from build123d import *

# Parameters (mm, degrees)
F1_DEPTH = 12.7
F2_DEPTH = 13.0175
F3_DEPTH = 12.065
F4_DEPTH = 13.0175
F5_DEPTH = 13.0175
F6_DEPTH = 12.7


with BuildPart() as f1:
    # F0 (on Front) → F1 (new body, symmetric)
    with BuildSketch(Plane.XZ):
        Polygon((28.078623, 2.014946), (28.042302, 12.433615), (27.101992, 12.433615), (27.101992, 12.053489), (26.661847, 12.053489), (26.661847, 12.433615), (22.280401, 12.433615), (20.983042, 11.892567), (21.152996, 9.532103), (23.8156, 7.73815), (23.8156, 6.359639), (23.060251, 5.60429), (23.060251, 2.620663), (24.042204, 2.035267), (24.042204, -0.005739), (25.287887, 0), (25.434768, 0.933369), (26.649874, 1.414069), (26.649874, 1.707831), (27.103869, 1.707831), (27.103869, 1.574303), align=None)
    extrude(amount=F1_DEPTH, both=True)

    # F0 (on Front) → F2 (join, symmetric)
    with BuildSketch(Plane.XZ):
        Polygon((20.983042, 11.892567), (22.280401, 12.433615), (22.003097, 12.804012), (14.739173, 12.804012), (3.162292, 11.001383), (-6.224729, 10.694268), (-7.46654, 9.492517), (-7.46654, 4.244864), (-7.106014, 4.244864), (-6.822593, 4.247176), (1.793046, 4.317466), (1.793046, 5.308367), (2.968092, 5.895891), (4.589082, 5.333918), (4.597188, 4.340344), (7.655644, 4.365296), (8.564113, 5.307411), (15.015916, 5.307411), (15.015916, 3.14395), (15.015916, 2.14362), (15.015916, -0.047328), (24.042204, -0.005739), (24.042204, 2.035267), (23.060251, 2.620663), (23.060251, 5.60429), (23.8156, 6.359639), (23.8156, 7.73815), (21.152996, 9.532103), align=None)
    extrude(amount=F2_DEPTH, both=True)

    # F0 (on Front) → F3 (join, symmetric)
    with BuildSketch(Plane.XZ):
        Polygon((7.581856, 3.14395), (15.015916, 3.14395), (15.015916, 5.307411), (8.564113, 5.307411), (7.655644, 4.365296), (4.597188, 4.340344), (1.793046, 4.317466), (-6.822593, 4.247176), (-6.793687, 0.704036), (-0.741626, 0.753411), (0, 2.14362), (0, 3.08393), (2.920319, 3.08393), (2.920319, 2.14362), (4.060694, 0.683138), (5.001005, 0.683138), (6.721572, 3.14395), align=None)
    extrude(amount=F3_DEPTH, both=True)

    # F0 (on Front) → F4 (join, symmetric)
    with BuildSketch(Plane.XZ):
        Polygon((13.963961, 2.14362), (15.015916, 2.14362), (15.015916, 3.14395), (7.581856, 3.14395), (7.581856, 1.583435), (13.323751, 1.583435), align=None)
        Polygon((0, 3.08393), (0, 2.14362), (1.525989, 1.676405), (2.920319, 2.14362), (2.920319, 3.08393), align=None)
    extrude(amount=F4_DEPTH, both=True)

    # F0 (on Front) → F5 (join, symmetric)
    with BuildSketch(Plane.XZ):
        Polygon((1.793046, 5.308367), (1.793046, 4.317466), (4.597188, 4.340344), (4.589082, 5.333918), (2.968092, 5.895891), align=None)
    extrude(amount=F5_DEPTH, both=True)

    # F0 (on Front) → F6 (join, symmetric)
    with BuildSketch(Plane.XZ):
        Polygon((-6.879017, -0.148209), (15.015916, -0.047328), (15.015916, 2.14362), (13.963961, 2.14362), (13.323751, 1.583435), (7.581856, 1.583435), (7.581856, 3.14395), (6.721572, 3.14395), (5.001005, 0.683138), (4.060694, 0.683138), (2.920319, 2.14362), (1.525989, 1.676405), (0, 2.14362), (-0.741626, 0.753411), (-6.793687, 0.704036), (-6.822593, 4.247176), (-7.106014, 4.244864), (-7.346365, 3.870985), (-7.346365, 0.145553), align=None)
    extrude(amount=F6_DEPTH, both=True)


solid = f1.part
Geometry: final body of the model. Coordinates: model frame, mm. A direction names the side the tool comes from. Round coordinates to 2 decimals unless told otherwise and drop trailing zeros. Loops run counter-clockwise (first coordinate to the right, second up) from the corner with the lowest first, then second, coordinate; pieces in that order, holes last. Notation, with made-up numbers: M 37,-15.75 L 70,-15.75 A21 cw 70,22.25 Z; hole C 67,-36 d4. An arc over 180 degrees is marked long. Put each result on its own line as item: value. Start each with the question number.
(1) Set-up query: faces 4 (the face through (8.104, -12.548, 4.83)), 5 (the face through (3.5, 12.4, 1.4)), 6 (the face through (25, 12.7, 8)). Return all of +Z, -Z, +X, -X, +Y, -Y with unobstructed straight access to the full face (end or side cutting, diameter ignored); none if empty.
(2) Material intervals for line 1 along Y through (x, z) = (26.5, 7.5); line 2 along Z through (x, y) = (22, -0.5); line 3 along Z through (x, y) = (24, 7.75), sorted ascending. Write a range as [from, to].
(3) Section query A-A (y = -5.75). Return loops of the section in (x, z).
(4) Contact query for flat-ended pins moving along their axis: pin 1 Ø1 at (x, y) = (11, -9.5) entering from +Z; pin 2 Ø3 at (y, z) = (3, 11) entering from +X; pin 3 Ø1.3 at (x, z) = (-1.5, 2) entering from +Y (3 decimals). Output: stop coordinate, or through.
(5) Draft query along Z for faces 1 (the face through (-7.346, 0, 2)), 2 (the face through (-6.84, -0.18, 10.1)), 3 (the face through (2.92, 12.5, 2.6)). Return one class per face: +Z half, -Z half, draft (parallel to the pull), parting line (faces both ways), or undercut.
Findings below:
1. face 4: -Y
1. face 5: +Y
1. face 6: +X, +Y
2. line 1: y = [-12.7, 12.7]
2. line 2: z = [-0.02, 12.8]
2. line 3: z = [-0.01, 12.43]
3. outline: M -7.47,4.24 L -7.11,4.24 L -7.35,3.87 L -7.35,0.15 L -6.88,-0.15 L 24.04,-0.01 L 25.29,0 L 25.43,0.93 L 26.65,1.41 L 26.65,1.71 L 27.1,1.71 L 27.1,1.57 L 28.08,2.01 L 28.04,12.43 L 27.1,12.43 L 27.1,12.05 L 26.66,12.05 L 26.66,12.43 L 22.28,12.43 L 22,12.8 L 14.74,12.8 L 3.16,11 L -6.22,10.69 L -7.47,9.49 Z
4. pin 1: stops at z = 12.3
4. pin 2: stops at x = 28.05
4. pin 3: stops at y = 12.065
5. face 1: draft
5. face 2: +Z half
5. face 3: undercut
